The listing builds one solid part. Answer for the finished solid, in the listing's coordinates (mm). A direction names the side the tool comes from. Give positions to 0.01 mm unless a question says otherwise; leave off trailing zeros. Loops run counter-clockwise (first coordinate to the right, second up) from the corner with the lowest first, then second, coordinate; pieces in that order, holes last. Notation, with made-up numbers: M 34,66 L 61,66 A30 cw 61,93 Z; hole C 46.5,89 d5. An arc over 180 degrees is marked long. Return JSON: item names as keys, results as strings.
Autodesk Inventor part; units mm, degrees
ref_plane "YZ Plane" through (0, 0, 0) normal (1, 0, 0) x (0, 1, 0)
ref_plane "XZ Plane" through (0, 0, 0) normal (0, 1, 0) x (-1, 0, 0)
ref_plane "XY Plane" through (0, 0, 0) normal (0, 0, 1) x (1, 0, 0)
sketch "Sketch1" plane through (0, 0, 0) normal (0, 0, 1) x (1, 0, 0)
  line L0 (0, 0) -> (0, 22)
  line L1 (0, 22) -> (32, 22)
  line L2 (32, 22) -> (32, 0)
  line L3 (32, 0) -> (0, 0)
  line L4 (16, 22) -> (16, 0) construction
  line L5 (32, 11) -> (0, 11) construction
  point P0 (3.5, 3.5)
  point P1 (28.5, 3.5)
  point P2 (3.5, 19.5)
  point P3 (28.5, 19.5)
  dimension "d0" = 32
  dimension "d1" = 22
  dimension "d2" = 3.5
  dimension "d3" = 3.5
  dimension "d4" = 2.5
extrude "Extrusion1" add sketch "Sketch1" against normal blind 8
hole "Hole1" at (3.5, 3.5, 0) at (28.5, 3.5, 0) at (3.5, 19.5, 0) at (28.5, 19.5, 0) direction (0, 0, -1) diameter 2.3813 depth 10 tip angle 118 countersink diameter 4 countersink angle 90
sketch "Sketch2" plane through (0, 0, -8) normal (0, 0, -1) x (-1, 0, 0)
  line L0 (-5.5, 1.75) -> (-26.5, 1.75)
  line L1 (-26.5, 1.75) -> (-26.5, 20.25)
  line L2 (-26.5, 20.25) -> (-5.5, 20.25)
  line L3 (-5.5, 20.25) -> (-5.5, 1.75)
  line L4 (-5.5, 1.75) -> (-26.5, 20.25) construction
  line L5 (-26.5, 1.75) -> (-5.5, 20.25) construction
  line L6 (-32, 22) -> (0, 22)
  line L7 (-16, 22) -> (-16, 0) construction
  line L8 (0, 0) -> (-32, 0)
  line L9 (-32, 0) -> (-32, 22)
  line L10 (-32, 11) -> (0, 11) construction
  line L11 (0, 22) -> (0, 0)
  point P0 (-16, 11)
  dimension "d14" = 21
  dimension "d15" = 18.5
extrude "Extrusion2" cut sketch "Sketch2" against normal blind 3.5 contours L0 L1 L2 L3
sketch "Sketch3" plane through (0, 0, -8) normal (0, 0, -1) x (-1, 0, 0)
  point P0 (0, 0)
properties part number "sensor_Mount"
(1) The part is cut by section D-D (x = 11.5). Determine the outline of the cut face in (y, z).
Values follow:
{"outline": "M 0,-8 L 1.75,-8 L 1.75,-4.5 L 20.25,-4.5 L 20.25,-8 L 22,-8 L 22,0 L 0,0 Z"}
(2) The part is cut by section C-C (z = -4). Determine the outline of the cut face in (x, y), and give its area (3 significant figures).
Values follow:
{"outline": "M 0,0 L 32,0 L 32,22 L 0,22 Z; hole C 3.5,3.5 d2.38; hole C 3.5,19.5 d2.38; hole C 28.5,3.5 d2.38; hole C 28.5,19.5 d2.38", "area": "686 mm²"}
(3) Given pin 1 (3 mm diameter, centred on x = 28.5, y = 19.5, fed in from +Z); pin 2 (1.4 mm diameter, centred on x = 3.5, y = 3.5, fed in from -Z); pin 3 (2.5 mm diameter, centred on x = 3.5, y = 19.5, fed in from +Z), each flat-ended and moving along its own axis, determine where each tip first touches the part or whether it passes through.
Values follow:
{"pin 1": "z = -0.5", "pin 2": "through", "pin 3": "z = -0.75"}
(4) The part is cut by section B-B (x = 3.5). Determine the outline of the cut face in (y, z), and give its area (3 significant figures).
Values follow:
{"outline": "M 0,-8 L 2.31,-8 L 2.31,-0.81 L 1.5,0 L 0,0 Z; M 4.69,-8 L 18.31,-8 L 18.31,-0.81 L 17.5,0 L 5.5,0 L 4.69,-0.81 Z; M 20.69,-8 L 22,-8 L 22,0 L 21.5,0 L 20.69,-0.81 Z", "area": "137 mm²"}
(5) Determine the mould class of faces 3 (the flat face through (16, 11, 0)), 4 (the flat face through (32, 11, -4)), 5 (the flat face through (16, 1.75, -6)) for opening direction X: released by +X, released by -X, zero draft, split by the parting line, or undercut.
Values follow:
{"face 3": "zero draft", "face 4": "released by +X", "face 5": "undercut"}
(6) Straight lines are drawn through the part: line 1 along X through (y, z) = (19.5, -3); line 2 along X through (y, z) = (19.5, -5.25); line 3 along Y through (x, z) = (11, -5). For each, find the intervals that lie inside material, in ascending order.
Values follow:
{"line 1": "0 to 2.31, 4.69 to 27.31, 29.69 to 32", "line 2": "0 to 2.31, 4.69 to 5.5, 26.5 to 27.31, 29.69 to 32", "line 3": "0 to 1.75, 20.25 to 22"}
(7) A tool of negligible diameter and unlimited length cuts with its end or side. For faces 1 (the flat face through (26.5, 11, -6)), 2 (the cylindrical face through (4.556, 2.951, -4.455)), from which of +Z, -Z, +X, -X, +Y, -Y can it reach the whole face along a straight path? Write none if from no direction.
Values follow:
{"face 1": "-Z", "face 2": "+Z, -Z"}
(8) The part is cut by section A-A (y = 3.5). Determine the outline of the cut face in (x, z).
Values follow:
{"outline": "M 0,-8 L 2.31,-8 L 2.31,-0.81 L 1.5,0 L 0,0 Z; M 4.69,-8 L 5.5,-8 L 5.5,-4.5 L 26.5,-4.5 L 26.5,-8 L 27.31,-8 L 27.31,-0.81 L 26.5,0 L 5.5,0 L 4.69,-0.81 Z; M 29.69,-8 L 32,-8 L 32,0 L 30.5,0 L 29.69,-0.81 Z"}
